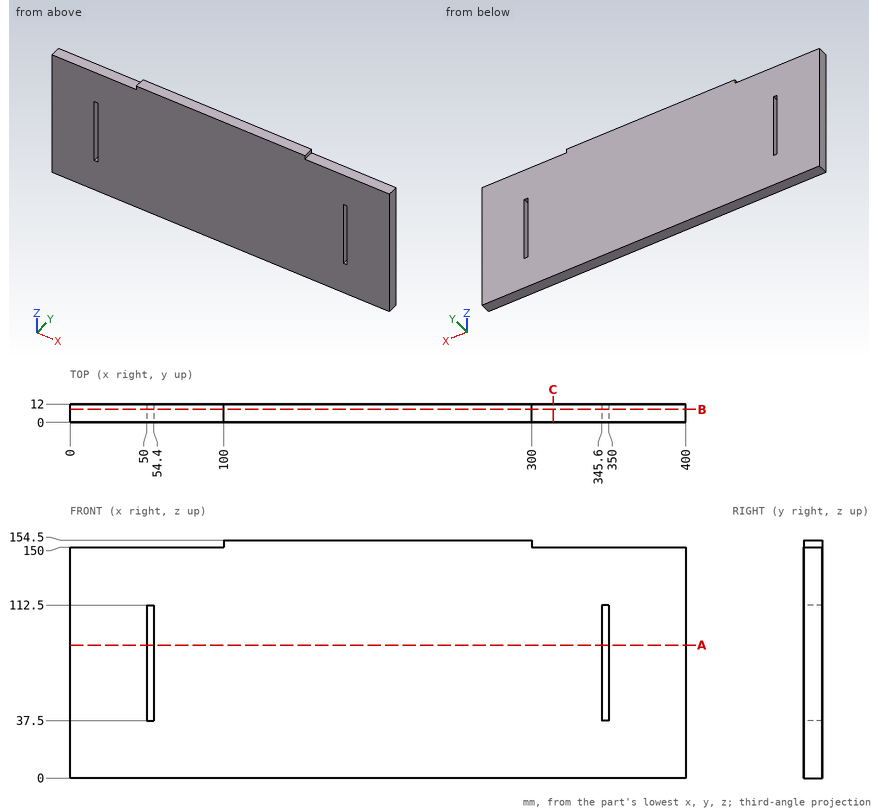
Here's the drawing with two shaded views (mm, measured from the low corner). I have some questions. Coordinates: 2 decimals unless noted, no trailing zeros. Loops run counter-clockwise (first coordinate to the right, second up) from the corner with the lowest first, then second, coordinate; pieces in that order, holes last. Notation, with made-up numbers: M -20.75,16.5 L 33.25,16.5 A35 ccw 33.25,49.5 Z; hole C 17.5,31 d7. An arc over 180 degrees is marked long. Return JSON: item names as keys, results as strings. Group by question number.
Item 1: Imagine slicing it at B-B (y = 8.5). Please give me the cut outline in (x, z).
Item 2: Imagine slicing it at A-A (z = 86.5). Please give me the cut outline in (x, y), and give its area (3 significant figures).
Item 3: If I drill on L1, parallel to X at y = 6, z = 96; L2, parallel to Z at x = 326, y = 8, over which ranges is the centre line in solid material (lowest first)? Write a range as from..to.
Item 4: Imagine slicing it at C-C (x = 314). Please give me the cut outline in (y, z), and give its area (3 significant figures).
Item 5: I'm going to push flat-ended pins straight in: pin 1 Ø3.5 at (x, y) = (64, 8.5) entering from +Z; pin 2 Ø1.3 at (y, z) = (7.5, 152.5) entering from +X. Where does each tip first touch, or does it pass through?
Verdict:
{
 "1": {"outline": "M 0,0 L 400,0 L 400,150 L 300,150 L 300,154.5 L 100,154.5 L 100,150 L 0,150 Z; hole M 50,37.5 L 54.4,37.5 L 54.4,112.5 L 50,112.5 Z; hole M 345.6,37.5 L 350,37.5 L 350,112.5 L 345.6,112.5 Z"},
 "2": {"outline": "M 0,0 L 50,0 L 50,12 L 0,12 Z; M 54.4,0 L 345.6,0 L 345.6,12 L 54.4,12 Z; M 350,0 L 400,0 L 400,12 L 350,12 Z", "area": "4,690 mm^2"},
 "3": {"L1": "x = 0..50, 54.4..345.6, 350..400", "L2": "z = 0..150"},
 "4": {"outline": "M 0,0 L 12,0 L 12,150 L 0,150 Z", "area": "1,800 mm^2"},
 "5": {"pin 1": "stops at z = 150", "pin 2": "stops at x = 300"}
}
